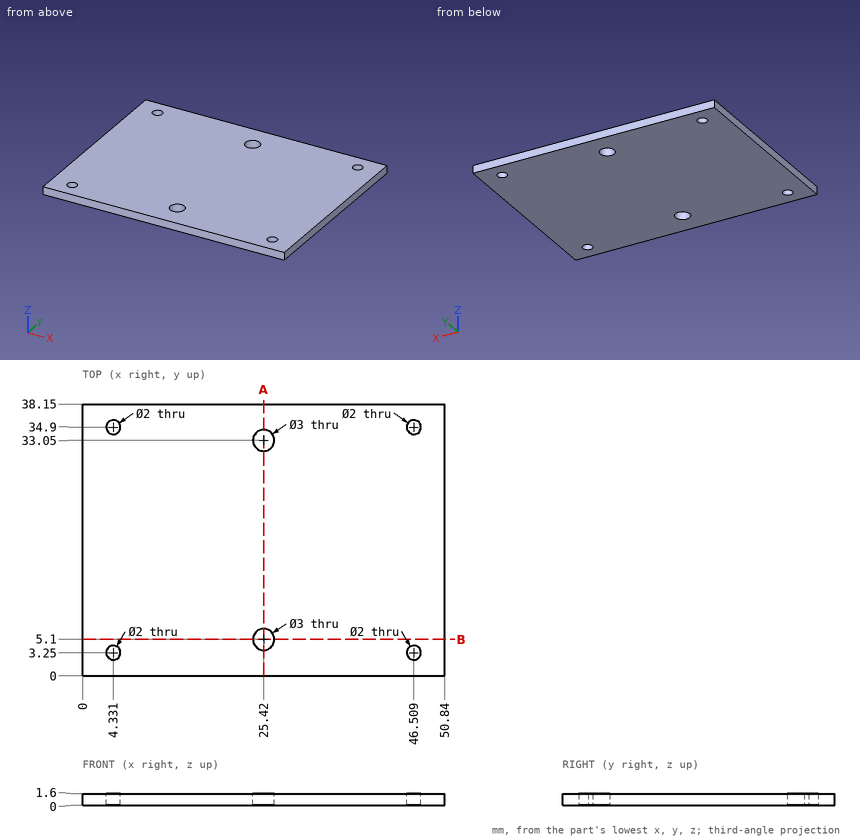
Answer from the drawing. Dimensions are ordinates in mm from the lowest x, y and z of the part. Give positions to 0.01 mm unless a question says otherwise; leave off trailing zeros. Loops run counter-clockwise (first coordinate to the right, second up) from the corner with the lowest first, then second, coordinate; pieces in that order, holes last.
Item 1: Find the intervals of material crossed by line 1 along Y through (x, z) = (25.42, 0.6); line 2 along X through (y, z) = (5.1, 0.45); line 3 along X through (y, z) = (34, 0.7) (1 decimal), in increasing order.
Derived:
line 1: y = 0 to 3.6, 6.6 to 31.55, 34.55 to 38.15
line 2: x = 0 to 23.92, 26.92 to 50.84
line 3: x = 0 to 3.9, 4.8 to 24.3, 26.6 to 46.1, 46.9 to 50.8
Item 2: A cutting plane is placed at A-A (x = 25.42). Give the vertices of the cut face in (y, z).
Derived:
outline: (0, 0) - (3.6, 0) - (3.6, 1.6) - (0, 1.6) - close; (6.6, 0) - (31.55, 0) - (31.55, 1.6) - (6.6, 1.6) - close; (34.55, 0) - (38.15, 0) - (38.15, 1.6) - (34.55, 1.6) - close
Item 3: This flat-tipped pin is pushed along its axis until it touches: pin 1 Ø6 at (x, y) = (9.5, 18) entering from -Z. Where does it stop, or does it pass through?
Derived:
pin 1: stops at z = 0
Item 4: A cutting plane is placed at B-B (y = 5.1). Give the vertices of the cut face in (x, z).
Derived:
outline: (0, 0) - (23.92, 0) - (23.92, 1.6) - (0, 1.6) - close; (26.92, 0) - (50.84, 0) - (50.84, 1.6) - (26.92, 1.6) - close
